Geometry check sheet. Reference: the model listing, model coordinates, mm. Coordinates: 2 decimals unless noted, no trailing zeros. Write each loop counter-clockwise with the first axis right and the second up, starting at its lowest first coordinate (ties: lowest second). Pieces come first, ordered by that corner, then holes. Notation, with made-up numbers: M 10.25,6.5 L 62.25,6.5 A32 cw 62.25,32.5 Z; hole C -17.5,74 d10. An arc over 180 degrees is marked long. Write item = value, one per line. Start each with the question number.
```python
from build123d import *

# Parameters (mm, degrees)
F0_R     = 38.1
F1_DEPTH = 38.1
F2_R     = 38.1
F3_DEPTH = 44.704
F4_R     = 38.1
F5_DEPTH = 63.246


with BuildPart() as f1:
    # F0 (on Front) → F1 (new body, symmetric)
    with BuildSketch(Plane.XZ):
        Circle(F0_R)
    extrude(amount=F1_DEPTH, both=True)

    # F2 (on Top) → F3 (intersect, symmetric)
    with BuildSketch(Plane.XY):
        Circle(F2_R)
    extrude(amount=F3_DEPTH, both=True, mode=Mode.INTERSECT)

    # F4 (on Right) → F5 (intersect, symmetric)
    with BuildSketch(Plane.YZ):
        Circle(F4_R)
    extrude(amount=F5_DEPTH, both=True, mode=Mode.INTERSECT)


solid = f1.part
```
Q1. Scan lines: L1, parallel to Y at x = -14, z = 17; L2, parallel to X at y = -10, z = 25.5; L3, parallel to X at y = 12.5, z = -26. Record each from-to range of solid material in increasing order.
Q2. Cross-section at C-C on z = -29.5. Enter the section's corners in (x, y), and give its area (3 significant figures).
Q3. Cross-section at A-A on y = -3. Enter the section's corners in (x, z).
Q4. Gauge pin test, flat ends, axial feed: pin 1 (4 mm diameter, centred on x = -18.5, z = -8, fed in from -Y); pin 2 (10 mm diameter, centred on x = 25.5, z = 1.5, fed in from -Y); pin 3 (2 mm diameter, centred on x = 8.5, z = -12, fed in from -Y). Record the tip position at first contact, or that the pin passes through.
Q5. Cross-section at B-B on x = 24.5. Enter the section's corners in (y, z), and give its area (3 significant figures).
Values found:
q1.L1 = -34.1 to 34.1
q1.L2 = -28.31 to 28.31
q1.L3 = -27.85 to 27.85
q2.outline = M -24.11,-24.11 L 24.11,-24.11 L 24.11,24.11 L -24.11,24.11 Z
q2.area = 2,330 mm²
q3.outline = M -37.98,-3 A38.1 ccw -3,-37.98 L 3,-37.98 A38.1 ccw 37.98,-3 L 37.98,3 A38.1 ccw 3,37.98 L -3,37.98 A38.1 ccw -37.98,3 Z
q4.pin_1 = -34.34
q4.pin_2 = -32.11
q4.pin_3 = -36.48
q5.outline = M -29.18,-24.5 A38.1 ccw -24.5,-29.18 L 24.5,-29.18 A38.1 ccw 29.18,-24.5 L 29.18,24.5 A38.1 ccw 24.5,29.18 L -24.5,29.18 A38.1 ccw -29.18,24.5 Z
q5.area = 3,360 mm²
